```python
from build123d import *

# Parameters (mm, degrees)
SKETCH2_W           = 1117.6
SKETCH2_H           = 2438.4
BOSS_EXTRUDE1_DEPTH = 736.6
CUT_EXTRUDE1_DEPTH  = 2439.4


with BuildPart() as part:
    # Sketch2 → Boss-Extrude1 (new body)
    with BuildSketch(Plane(origin=(0, 0, 0), x_dir=(1, 0, 0), z_dir=(0, 1, 0))):
        Rectangle(SKETCH2_W, SKETCH2_H)
    extrude(amount=BOSS_EXTRUDE1_DEPTH)

    # Sketch3 → Cut-Extrude1 (cut, through all)
    with BuildSketch(Plane.XY.offset(1219.2)):
        with BuildLine():
            Line((-148.287166209, 109.524357008), (-148.287166209, 286.88743816))
            ThreePointArc((-148.287166209, 286.88743816), (-268.523591462, 577.163846698), (-558.8, 697.400271951))
            Line((-558.8, 697.400271951), (-558.8, 0))
            Line((-558.8, 0), (-481.206392305, 0))
            Line((-481.206392305, 0), (-481.206392305, 29.565590915))
            Line((-481.206392305, 29.565590915), (-148.287166209, 109.524357008))
        make_face()
        with BuildLine():
            Line((558.8, 0), (481.206392305, 0))
            Line((481.206392305, 0), (481.206392305, 29.565590915))
            Line((481.206392305, 29.565590915), (148.287166209, 109.524357008))
            Line((148.287166209, 109.524357008), (148.287166209, 286.88743816))
            ThreePointArc((148.287166209, 286.88743816), (268.523591462, 577.163846698), (558.8, 697.400271951))
            Line((558.8, 697.400271951), (558.8, 0))
        make_face()
    extrude(amount=-CUT_EXTRUDE1_DEPTH, mode=Mode.SUBTRACT)


solid = part.part
```
Work out the finished part from the listing and answer in its coordinate system (mm). A direction names the side the tool comes from. Give positions to 0.01 mm unless a question says otherwise; leave off trailing zeros. Loops run counter-clockwise (first coordinate to the right, second up) from the corner with the lowest first, then second, coordinate; pieces in that order, holes last. Notation, with made-up numbers: (25, 16) -> (58, 16) arc R19 ccw to (58, 21) -> close; hole circle Ø10 at (69.25, 40). An arc over 180 degrees is marked (long way). One line per question, with ' | ' between items. Start each with the question number.
1) Section B-B, the plane x = 312 is taken. Determine the outline of the cut face in (y, z), then the cut area to 3 significant figures.
2) For faces 4 (the face through (-8, 363, -1219.2)), 5 (the face through (-317.077, 68.985, 17.069)), 6 (the face through (265.349, 573.955, 17.069)), determine the directions among +Z, -Z, +X, -X, +Y, -Y from which every point of the face is accessible in a straight line to the end or side of a thin tool.
3) Section C-C, the plane y = 179 is taken. Determine the outline of the cut face in (x, z).
4) Section A-A, the plane z = -963 is taken. Determine the outline of the cut face in (x, y).
5) Section D-D, the plane y = 466.5 is taken. Determine the outline of the cut face in (x, z), then the cut area to 3 significant figures.
6) Straight lines are drawn through the part: L1, parallel to X at y = 170, z = 769.5; L2, parallel to Y at x = -282.5, z = 299; L3, parallel to Y at x = -288, z = -927.5. For each, find the intervals that lie inside material, in ascending order.
7) Determine the mould class of faces 1 (the face through (-7, 0, -17)), 2 (the face through (-8, 736.6, -17)), 3 (the face through (148.287, 197, 17)) for opening direction Y: +Y half, -Y half, draft (parallel to the pull), parting line (faces both ways), or undercut.
8) Each of these flat-tipped pins is pushed along its axis until it touches: pin 1 (15 mm diameter, centred on y = 8.5, z = -590.5, fed in from +X); pin 2 (23.5 mm diameter, centred on y = 14.5, z = -17, fed in from -X); pin 3 (8 mm diameter, centred on y = 227.5, z = -301, fed in from +X). Where does it stop, or does it pass through?
Resolved:
1) outline: (0, -1219.2) -> (70.2, -1219.2) -> (70.2, 1219.2) -> (0, 1219.2) -> close; (614.93, -1219.2) -> (736.6, -1219.2) -> (736.6, 1219.2) -> (614.93, 1219.2) -> close | area: 468,000 mm2
2) face 4: -Z, +X, -X, +Y, -Y | face 5: +Z, -Z, -X | face 6: +Z, -Z, +X
3) outline: (-148.29, -1219.2) -> (148.29, -1219.2) -> (148.29, 1219.2) -> (-148.29, 1219.2) -> close
4) outline: (-558.8, 697.4) arc R410.51 cw to (-148.29, 286.89) -> (-148.29, 109.52) -> (-481.21, 29.57) -> (-481.21, 0) -> (481.21, 0) -> (481.21, 29.57) -> (148.29, 109.52) -> (148.29, 286.89) arc R410.51 cw to (558.8, 697.4) -> (558.8, 736.6) -> (-558.8, 736.6) -> close
5) outline: (-189.67, -1219.2) -> (189.67, -1219.2) -> (189.67, 1219.2) -> (-189.67, 1219.2) -> close | area: 925,000 mm2
6) L1: -148.29 to 148.29 | L2: 0 to 77.29, 590.5 to 736.6 | L3: 0 to 75.97, 595.41 to 736.6
7) face 1: -Y half | face 2: +Y half | face 3: undercut
8) pin 1: x = 481.21 | pin 2: x = -481.21 | pin 3: x = 148.29
